The listing builds one solid part. Answer for the finished solid, in the listing's coordinates (mm). A direction names the side the tool comes from. Coordinates: 2 decimals unless noted, no trailing zeros. Order: outer loops, then holes, each group sorted by start corner. A loop starts at its lowest first (then second) coordinate and runs counter-clockwise, first axis right, second up. Notation, with made-up numbers: (60, -33) -> (69, -33) arc R22 ccw to (69, -2) -> close; hole circle Ø9 at (65.5, 37.5). An arc over 180 degrees is marked (long way). Return JSON: item names as keys, results as strings.
from build123d import *

# Parameters (mm, degrees)
F1_DEPTH    = 6.35
F2_T1_DEPTH = 6.35
F3_D        = 14.2875


# Not quite as in the source:
# - a fillet or chamfer that OpenCascade refuses, or shapes differently, is made with other operations: its cross-section is extruded or revolved along the edge and cut away or added
# - a length typed as a fraction of an inch, garbled in the dataset ("3 / 203.2 mm" for 3/8 in), is restored


with BuildPart() as f1:
    # F0 (on Top) → F1 (new body)
    with BuildSketch(Plane.XY):
        with BuildLine():
            Line((-81.6372310897, 19.05), (-85.725, 19.05))
            Line((-85.725, 19.05), (-85.725, -19.05))
            Line((-85.725, -19.05), (-39.5493225013, -19.05))
            Line((-39.5493225013, -19.05), (85.725, -19.05))
            Line((85.725, -19.05), (85.725, 19.05))
            Line((85.725, 19.05), (81.6372310897, 19.05))
            ThreePointArc((81.6372310897, 19.05), (66.2692873292, 12.0114502249), (50.3024058786, 6.4640566836))
            ThreePointArc((50.3024058786, 6.4640566836), (47.5991921402, 13.3341571472), (42.9264215083, 19.05))
            Line((42.9264215083, 19.05), (11.0735784917, 19.05))
            ThreePointArc((11.0735784917, 19.05), (4.806476702, 10.0660406788), (3.2107124888, -0.7710081124))
            ThreePointArc((3.2107124888, -0.7710081124), (0, -0.8), (-3.2107124888, -0.7710081124))
            ThreePointArc((-3.2107124888, -0.7710081124), (-4.806476702, 10.0660406788), (-11.0735784917, 19.05))
            Line((-11.0735784917, 19.05), (-42.9264215083, 19.05))
            ThreePointArc((-42.9264215083, 19.05), (-47.5991921402, 13.3341571472), (-50.3024058786, 6.4640566836))
            ThreePointArc((-50.3024058786, 6.4640566836), (-66.2692873292, 12.0114502249), (-81.6372310897, 19.05))
        make_face()
        with BuildLine():
            ThreePointArc((-11.0735784917, 19.05), (-27, 25.1380132129), (-42.9264215083, 19.05))
            Line((-42.9264215083, 19.05), (-11.0735784917, 19.05))
        make_face()
        with BuildLine():
            ThreePointArc((42.9264215083, 19.05), (27, 25.1380132129), (11.0735784917, 19.05))
            Line((11.0735784917, 19.05), (42.9264215083, 19.05))
        make_face()
    extrude(amount=F1_DEPTH)

    # F2: fillet of radius 3.175 on 4 edges, made by hand

    # F2_s2 → F2_t1 (join)
    with BuildSketch(Plane.XY):
        with BuildLine():
            ThreePointArc((53.4010264507, 7.4088139849), (51.0383331441, 7.5920475012), (49.4606483484, 9.3603248744))
            ThreePointArc((49.4606483484, 9.3603248744), (49.9273063268, 7.9254958305), (50.3024058786, 6.4640566836))
            ThreePointArc((50.3024058786, 6.4640566836), (51.8538678481, 6.9293782301), (53.4010264507, 7.4088139849))
        make_face()
        with BuildLine():
            ThreePointArc((3.1442176475, 2.2443697426), (2.1701152487, 0.084041365), (-0.0286046325, -0.799997699))
            ThreePointArc((-0.0286046325, -0.799997699), (1.5911199519, -0.792880446), (3.2107124888, -0.7710081124))
            ThreePointArc((3.2107124888, -0.7710081124), (3.1298031747, 0.7356297793), (3.1442176475, 2.2443697426))
        make_face()
        with BuildLine():
            ThreePointArc((0.0286046325, -0.799997699), (-2.1701152487, 0.084041365), (-3.1442176475, 2.2443697426))
            ThreePointArc((-3.1442176475, 2.2443697426), (-3.1298031747, 0.7356297793), (-3.2107124888, -0.7710081124))
            ThreePointArc((-3.2107124888, -0.7710081124), (-1.5911199519, -0.792880446), (0.0286046325, -0.799997699))
        make_face()
        with BuildLine():
            ThreePointArc((-53.4010264507, 7.4088139849), (-51.0383331441, 7.5920475012), (-49.4606483484, 9.3603248744))
            ThreePointArc((-49.4606483484, 9.3603248744), (-49.9273063268, 7.9254958305), (-50.3024058786, 6.4640566836))
            ThreePointArc((-50.3024058786, 6.4640566836), (-51.8538678481, 6.9293782301), (-53.4010264507, 7.4088139849))
        make_face()
    extrude(amount=F2_T1_DEPTH)

    # F3 (through all)
    with Locations(Plane(origin=(0, 0, 0), x_dir=(1, 0, 0), z_dir=(0, 0, -1))):
        with Locations((-69.088, 0), (-27, -1.2620132129), (27, -1.2620132129), (69.088, 0)):
            Hole(F3_D / 2)


solid = f1.part
1. Consider line 1 (X direction, y = -1, z = 3) (3 decimals); line 2 (Y direction, x = -27, z = 2.5); line 3 (X direction, y = 13.5, z = 4.5) (3 decimals). Determine where each line is inside the solid, lowest interval first. Write a range as from..to.
Answer block:
{"line 1": "x = -85.725..-76.161, -62.015..-33.776, -20.224..20.224, 33.776..62.015, 76.161..85.725", "line 2": "y = -19.05..-5.88, 8.41..25.14", "line 3": "x = -85.725..-69.861, -47.501..-6.499, 6.499..47.501, 69.861..85.725"}
2. The part is cut by section A-A on x = 27. Give the vertices of the cut face in (y, z), and give its area (3 significant figures).
Answer block:
{"outline": "(-19.05, 0) -> (-5.88, 0) -> (-5.88, 6.35) -> (-19.05, 6.35) -> close; (8.41, 0) -> (25.14, 0) -> (25.14, 6.35) -> (8.41, 6.35) -> close", "area": "190 mm2"}
3. This flat-tipped pin is pushed along its axis until it touches: pin 1 Ø2 at (x, z) = (-84.5, 2.5) entering from +Y. Where does it stop, or does it pass through?
Answer block:
{"pin 1": "stops at y = 19.05"}
4. The part is cut by section B-B on z = 4.5. Give the number of separate pieces and of enclosed holes in the cut face, and give its area (3 significant figures).
Answer block:
{"separate pieces": "1", "enclosed holes": "4", "area": "5,450 mm2"}
5. The part is cut by section D-D on x = -51.5. Give the vertices of the cut face in (y, z).
Answer block:
{"outline": "(-19.05, 0) -> (7.41, 0) -> (7.41, 6.35) -> (-19.05, 6.35) -> close"}
6. For faces 1 (the face through (2.205, 0.118, 3.131)), 2 (the face through (-84, 19.05, 3)), 3 (the face through (84, 19.05, 3)), determine the directions among +Z, -Z, +X, -X, +Y, -Y from which every point of the face is accessible in a straight line to the end or side of a thin tool.
Answer block:
{"face 1": "+Z, -Z, +Y", "face 2": "+Z, -Z, -X, +Y", "face 3": "+Z, -Z, +X, +Y"}
7. The part is cut by section C-C on x = 71. Give the vertices of the cut face in (y, z).
Answer block:
{"outline": "(-19.05, 0) -> (-6.88, 0) -> (-6.88, 6.35) -> (-19.05, 6.35) -> close; (6.88, 0) -> (13.99, 0) -> (13.99, 6.35) -> (6.88, 6.35) -> close"}
